Source: CAD feature listing. Evaluate the final solid. Frame: model axes, mm. Face numbers are marked on the shaded views. Round coordinates to 2 decimals unless told otherwise and drop trailing zeros. Loops run counter-clockwise (first coordinate to the right, second up) from the corner with the lowest first, then second, coordinate; pieces in that order, holes last. Notation, with made-up numbers: (-35, 5) - (-13, 5) arc R13 ccw to (-13, 10) - close; hole circle Ø9 at (-8.75, 2.25). An arc over 180 degrees is marked (long way). Use CSV: the item, a comma, the result in double quotes. Start each with the question number.
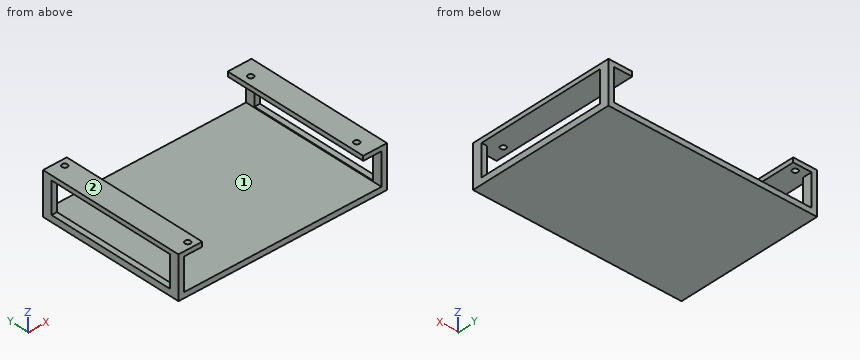
from build123d import *

# Parameters (mm, degrees)
SKETCH10_W              = 114
SKETCH10_H              = 80
BOSS_EXTRUDE6_DEPTH     = 3
SKETCH12_W              = 3
SKETCH12_H              = 80
BOSS_EXTRUDE7_DEPTH     = 20
SKETCH13_W              = 2.5
SKETCH13_H              = 80
BOSS_EXTRUDE8_DEPTH     = 10
SKETCH16_W              = 16
SKETCH16_H              = 70
CUT_EXTRUDE3_DEPTH      = 135.434200024
SKETCH18_R              = 1.5
CUT_EXTRUDE4_DEPTH      = 10
CUT_EXTRUDE5_DEPTH      = 132.899788234
CUT_EXTRUDE5_DEPTH_BACK = 132.899788234
SKETCH19_W              = 1
SKETCH19_H              = 70


with BuildPart() as part:
    # Sketch10 → Boss-Extrude6 (new body)
    with BuildSketch(Plane.XY):
        with Locations((23.926213283, 27.43555543)):
            Rectangle(SKETCH10_W, SKETCH10_H)
    extrude(amount=BOSS_EXTRUDE6_DEPTH)

    # Sketch12 → Boss-Extrude7 (add)
    with BuildSketch(Plane.XY.offset(3)):
        with Locations((-31.573786717, 27.43555543)):
            Rectangle(SKETCH12_W, SKETCH12_H)
    boss_extrude7 = extrude(amount=BOSS_EXTRUDE7_DEPTH)

    # Sketch13 → Boss-Extrude8 (add)
    with BuildSketch(Plane(origin=(-30.073786717, 0, 0), x_dir=(0, 0, -1), z_dir=(1, 0, 0))):
        with Locations((-21.75, 27.43555543)):
            Rectangle(SKETCH13_W, SKETCH13_H)
    boss_extrude8 = extrude(amount=BOSS_EXTRUDE8_DEPTH)

    # Mirror3: Boss-Extrude7, Boss-Extrude8 across plane
    add(boss_extrude7.mirror(Plane.ZY.offset(-23.926213283)))
    add(boss_extrude8.mirror(Plane.ZY.offset(-23.926213283)))

    # Sketch16 → Cut-Extrude3 (cut, through all)
    with BuildSketch(Plane.ZY.offset(33.073786717)):
        with Locations((11.5, 27.43555543)):
            Rectangle(SKETCH16_W, SKETCH16_H)
    extrude(amount=-CUT_EXTRUDE3_DEPTH, mode=Mode.SUBTRACT)

    # Sketch18 → Cut-Extrude4 (cut)
    with BuildSketch(Plane.XY.offset(23)):
        with Locations((-24.573786717, 63.728579771)):
            Circle(SKETCH18_R)
        with Locations((-24.573786717, -8.857468911)):
            Circle(SKETCH18_R)
        with Locations((72.426213283, 58.728579771)):
            Circle(SKETCH18_R)
        with Locations((72.426213283, -3.857468911)):
            Circle(SKETCH18_R)
    extrude(amount=-CUT_EXTRUDE4_DEPTH, mode=Mode.SUBTRACT)

    # Sketch19 → Cut-Extrude5 (cut, two sides: drawn at the far end of the back side and taken through both)
    with BuildSketch(Plane.ZY.offset(-77.926213283).offset(-CUT_EXTRUDE5_DEPTH_BACK)):
        with Locations((20, 27.43555543)):
            Rectangle(SKETCH19_W, SKETCH19_H)
    extrude(amount=CUT_EXTRUDE5_DEPTH + CUT_EXTRUDE5_DEPTH_BACK, mode=Mode.SUBTRACT)


solid = part.part
1. Mould query, pull axis X, two halves, no side actions, for the marked faces 1 and 2. Classes: +X half, -X half, draft (parallel to the pull), parting line (faces both ways), or undercut.
2. Line query: line 1 along Z through (x, y) = (16, 24.5); line 2 along Z through (x, y) = (-27.5, -8.5). Output: solid intervals per line, ascending.
3. Section query A-A on z = 10.5. Return the cut outline in (x, y).
4. Section query C-C on x = 45. Return the cut outline in (y, z), and give its area (3 significant figures).
5. Contact query for a flat-ended pin moving along its axis: P1, Ø1.8, axis at x = -24.57, y = 63.73, coming from the +Z side. Output: stop coordinate, or through.
6. Section query B-B on y = 47. Return the cut outline in (x, z), and give its area (3 significant figures).
Values:
1,face 1,"undercut"
1,face 2,"draft"
2,line 1,"z = 0 to 3"
2,line 2,"z = 0 to 3, 20.5 to 23"
3,outline,"(-33.07, -12.56) - (-30.07, -12.56) - (-30.07, -7.56) - (-33.07, -7.56) - close; (-33.07, 62.44) - (-30.07, 62.44) - (-30.07, 67.44) - (-33.07, 67.44) - close; (77.93, -12.56) - (80.93, -12.56) - (80.93, -7.56) - (77.93, -7.56) - close; (77.93, 62.44) - (80.93, 62.44) - (80.93, 67.44) - (77.93, 67.44) - close"
4,outline,"(-12.56, 0) - (67.44, 0) - (67.44, 3) - (-12.56, 3) - close"
4,area,"240 mm^2"
5,P1,"stops at z = 3"
6,outline,"(-33.07, 0) - (80.93, 0) - (80.93, 3.5) - (77.93, 3.5) - (77.93, 3) - (-30.07, 3) - (-30.07, 3.5) - (-33.07, 3.5) - close; (-33.07, 20.5) - (-20.07, 20.5) - (-20.07, 23) - (-33.07, 23) - close; (67.93, 20.5) - (80.93, 20.5) - (80.93, 23) - (67.93, 23) - close"
6,area,"410 mm^2"
